Geometry check sheet. Reference: the model listing, model coordinates, mm. A direction names the side the tool comes from. Round coordinates to 2 decimals unless told otherwise and drop trailing zeros. Order: outer loops, then holes, each group sorted by start corner. A loop starts at its lowest first (then second) coordinate and runs counter-clockwise, first axis right, second up. Notation, with made-up numbers: (22, 36.5) - (52, 36.5) arc R27 cw to (52, 54.5) - close; hole circle Ø2 at (32, 56). An arc over 180 degrees is marked (long way). Use a Markdown table: item, result. Add a question column.
(1) Access from +Z, -Z, +X, -X, +Y, -Y to the whole of each face (thin tool, end or side, straight path). Record for faces 1 (the face through (-23.3, -10.3, 28.8)), 2 (the face through (0, 0, 2)), 3 (the face through (-23.072, -10.1, 0.986)).
(2) Section check A-A on z = 6.5. Record the boundary of the cut face in (x, y).
(3) Gauge pin test, flat ends, axial feed: P1, Ø9.5, axis at x = -3.5, y = -1, coming from the +Z side; P2, Ø13, axis at x = -9, z = 20.5, coming from the -Y side. Record the tip position at first contact, or that the pin passes through.
(4) Thickness scan on line 1 along Y through (x, z) = (-21, 16); line 2 along X through (y, z) = (1.5, 12); line 3 along Z through (x, y) = (-1, -2.25). Record the ranges inside material, lowest first. Write a range as [from, to].
(5) Mould release check, pull along X, two halves, no side actions. Record for faces 4 (the face through (23.915, 0.853, 0.986)), 5 (the face through (23.5, 0.9, 29)), 6 (the face through (0, 11.5, 15)): released by +X, released by -X, zero draft, split by the parting line, or undercut.
(6) Section check D-D on z = 27. Record the boundary of the cut face in (x, y).
```python
from build123d import *

# Parameters (mm, degrees)
F0_W     = 49
F0_H     = 23
F1_DEPTH = 30
F2_T     = -2
F3_SIZE  = 1.99999
F5_DEPTH = 2
F6_SIZE  = 1.9999
F7_SIZE  = 1.99999
F8_SIZE2 = 1.1547005384
F8_SIZE  = 2


# Not quite as in the source:
# - a fillet or chamfer is up to 0.001 mm smaller than in the source, because OpenCascade refuses the exact size


with BuildPart() as f1:
    # F0 (on Top) → F1 (new body)
    with BuildSketch(Plane.XY):
        Rectangle(F0_W, F0_H)
    extrude(amount=F1_DEPTH)

    # F2
    f2_openings = [f1.faces().sort_by_distance(p)[0] for p in [
        (0, 0, 30),
    ]]
    offset(amount=F2_T, openings=f2_openings)

    # F3 (size 2 in the source; OpenCascade refuses exactly that, so slightly less here)
    f3_edges = [f1.edges().sort_by_distance(p)[0] for p in [
        (0, 9.5, 30),
        (-22.5, 0, 30),
        (22.5, 0, 30),
    ]]
    chamfer(f3_edges, length=F3_SIZE)

    # F4 (on face) → F5 (cut, through all)
    with BuildSketch(Plane.XZ.offset(11.5)):
        with BuildLine():
            Line((-22.5, 30), (-22.5, 28))
            ThreePointArc((-22.5, 28), (0, 17.843134833), (22.5, 28))
            Line((22.5, 28), (22.5, 30))
            Line((22.5, 30), (-22.5, 30))
        make_face()
    extrude(amount=-F5_DEPTH, mode=Mode.SUBTRACT)

    # F6 (size 2 in the source; OpenCascade refuses exactly that, so slightly less here)
    f6_edges = [f1.edges().sort_by_distance(p)[0] for p in [
        (-22.5, -10.5, 30),
        (22.5, -10.5, 30),
    ]]
    chamfer(f6_edges, length=F6_SIZE)

    # F7 (size 2 in the source; OpenCascade refuses exactly that, so slightly less here)
    f7_edges = [f1.edges().sort_by_distance(p)[0] for p in [
        (-24.5, -11.5, 15),
        (24.5, -11.5, 15),
    ]]
    chamfer(f7_edges, length=F7_SIZE)

    # F8
    f8_edges = [f1.edges().sort_by_distance(p)[0] for p in [
        (24.5, 0.999995, 0),
        (23.500005, -10.500005, 0),
        (0, -11.5, 0),
        (-23.500005, -10.500005, 0),
        (-24.5, 0.999995, 0),
    ]]
    chamfer(f8_edges, length=F8_SIZE, length2=F8_SIZE2)


solid = f1.part
```
Check sheet entries:
| question | item | result |
|---|---|---|
| 1 | face 1 | +Z, -Y |
| 1 | face 2 | +Z |
| 1 | face 3 | -Z, -X, -Y |
| 2 | outline | (-24.5, -9.5) - (-22.5, -11.5) - (22.5, -11.5) - (24.5, -9.5) - (24.5, 11.5) - (-24.5, 11.5) - close; hole (-22.5, -9.5) - (22.5, -9.5) - (22.5, 9.5) - (-22.5, 9.5) - close |
| 3 | P1 | stops at z = 2 |
| 3 | P2 | stops at y = -11.5 |
| 4 | line 1 | y = [-11.5, -9.5], [9.5, 11.5] |
| 4 | line 2 | x = [-24.5, -22.5], [22.5, 24.5] |
| 4 | line 3 | z = [0, 2] |
| 5 | face 4 | released by +X |
| 5 | face 5 | undercut |
| 5 | face 6 | zero draft |
| 6 | outline | (-24.5, -9.5) - (-22.5, -11.5) - (-21.58, -11.5) - (-21.58, -9.5) - (-22.5, -9.5) - (-22.5, 9.5) - (22.5, 9.5) - (22.5, -9.5) - (21.58, -9.5) - (21.58, -11.5) - (22.5, -11.5) - (24.5, -9.5) - (24.5, 11.5) - (-24.5, 11.5) - close |
